Could you check a few things on this model? Use its own coordinates, in mm. Round coordinates to 2 decimals unless told otherwise and drop trailing zeros. Put each result on its own line as item: value.
from build123d import *

# Parameters (mm, degrees)
SKETCH_1_R      = 2.55
EXTRUDE_1_DEPTH = 592.5


with BuildPart() as part:
    # Эскиз1 → Бобышка-Вытянуть1 (new body)
    with BuildSketch(Plane.XY.offset(792.9)):
        Polygon((-8.2, -3.125), (-8.506400721, -3.125), (-10, -4.58), (-10, -15.42), (-8.506400721, -16.875), (-8.2, -16.875), (-8.2, -14.5), (-7.00202244, -14.5), (-3.9, -17.521856474), (-3.9, -19.8), (-3.7, -20), (-3.9, -20.2), (-3.9, -22.478143526), (-7.00202244, -25.5), (-8.2, -25.5), (-8.2, -23.125), (-8.506400721, -23.125), (-10, -24.58), (-10, -30), (-4.58, -30), (-3.125, -28.506400721), (-3.125, -28.2), (-5.5, -28.2), (-5.5, -27.00202244), (-2.478143526, -23.9), (-0.2, -23.9), (0, -23.7), (0.2, -23.9), (2.478143526, -23.9), (5.5, -27.00202244), (5.5, -28.2), (3.125, -28.2), (3.125, -28.506400721), (4.58, -30), (10, -30), (10, -24.58), (8.506400721, -23.125), (8.2, -23.125), (8.2, -25.5), (7.00202244, -25.5), (3.9, -22.478143526), (3.9, -20.2), (3.7, -20), (3.9, -19.8), (3.9, -17.521856474), (7.00202244, -14.5), (8.2, -14.5), (8.2, -16.875), (8.506400721, -16.875), (10, -15.42), (10, -4.58), (8.506400721, -3.125), (8.2, -3.125), (8.2, -5.5), (7.00202244, -5.5), (3.9, -2.478143526), (3.9, -0.2), (3.7, 0), (3.9, 0.2), (3.9, 2.478143526), (7.00202244, 5.5), (8.2, 5.5), (8.2, 3.125), (8.506400721, 3.125), (10, 4.58), (10, 10), (4.58, 10), (3.125, 8.506400721), (3.125, 8.2), (5.5, 8.2), (5.5, 7.00202244), (2.478143526, 3.9), (0.2, 3.9), (0, 3.7), (-0.2, 3.9), (-2.478143526, 3.9), (-5.5, 7.00202244), (-5.5, 8.2), (-3.125, 8.2), (-3.125, 8.506400721), (-4.58, 10), (-10, 10), (-10, 4.58), (-8.506400721, 3.125), (-8.2, 3.125), (-8.2, 5.5), (-7.00202244, 5.5), (-3.9, 2.478143526), (-3.9, 0.2), (-3.7, 0), (-3.9, -0.2), (-3.9, -2.478143526), (-7.00202244, -5.5), (-8.2, -5.5), align=None)
        Circle(SKETCH_1_R, mode=Mode.SUBTRACT)
        with Locations((0, -20)):
            Circle(SKETCH_1_R, mode=Mode.SUBTRACT)
        Polygon((-2.478143526, -3.9), (2.478143526, -3.9), (5.5, -7.00202244), (8.2, -7.00202244), (8.2, -12.99797756), (5.5, -12.99797756), (2.478143526, -16.1), (-2.478143526, -16.1), (-5.5, -12.99797756), (-8.2, -12.99797756), (-8.2, -7.00202244), (-5.5, -7.00202244), align=None, mode=Mode.SUBTRACT)
    extrude(amount=-EXTRUDE_1_DEPTH)


solid = part.part
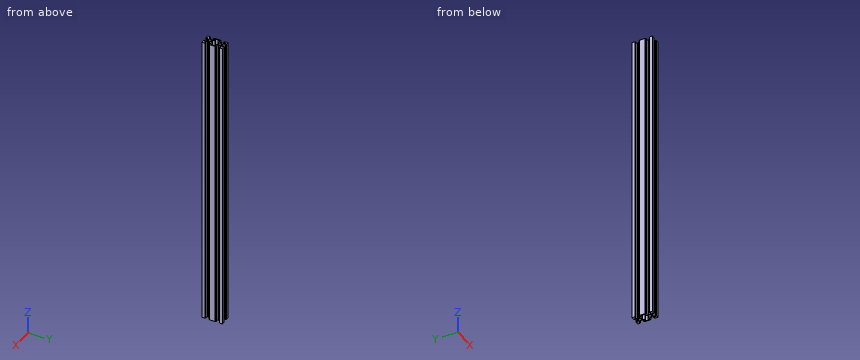
(1) Please list where these lines run through material, in increasing order: probe 1 along Y at (x, z) = (-8.25, 695) (3 decimals); probe 2 along Y at (x, z) = (0, 389.5); probe 3 along Y at (x, z) = (0.25, 287). Write a range as from..to.
Values found:
probe 1: y = -30..-23.125, -16.875..-3.125, 3.125..10
probe 2: y = -23.7..-22.55, -17.45..-16.1, -3.9..-2.55, 2.55..3.7
probe 3: y = -23.9..-22.54, -17.46..-16.1, -3.9..-2.54, 2.54..3.9
(2) I'm going to push flat-ended pins straight in: pin 1 (4 mm diameter, centred on x = -1, z = 601, fed in from +Y); pin 2 (1.1 mm diameter, centred on y = -22, z = 383, fed in from -X); pin 3 (1 mm diameter, centred on y = -17, z = 728, fed in from +X). Where does each tip first touch, or does it pass through?
Values found:
pin 1: stops at y = 4.44
pin 2: stops at x = -3.97
pin 3: stops at x = 8.89
(3) Imagine slicing it at A-A, the plane z = 574. Give the number of separate pieces and of enclosed holes in the cut face, then the cut area to 3 significant figures.
Values found:
separate pieces: 1
enclosed holes: 3
area: 303 mm^2
